Verification items for this drawing (mm, ordinates from the low corner). A direction names the side the tool comes from. Round coordinates to 2 decimals unless told otherwise and drop trailing zeros. Order: outer loops, then holes, each group sorted by start corner. A loop starts at its lowest first (then second) coordinate and runs counter-clockwise, first axis right, second up. Notation, with made-up numbers: (0, -28) - (33, -28) arc R10 ccw to (33, -14) - close; hole circle Ø1 at (-1, 38). An arc over 180 degrees is marked (long way). Return JSON: item names as keys, results as strings. Group by question number.
Q1. Sectioned sample at D-D, the plane x = 1.5. Record the cut outline in (y, z), then the cut area to 3 significant figures.
Q2. Sectioned sample at C-C, the plane y = 5. Record the cut outline in (x, z), then the cut area to 3 significant figures.
Q3. Tool access check on the marked faces 1 and 2. Record the directions out of +Z, -Z, +X, -X, +Y, -Y that give a thin tool (end or side, any length) a straight path to the whole face; none if there is none.
Q4. Material ranges on line 1 along Y through (x, z) = (7.5, 6.5); line 2 along Y through (x, z) = (5.25, 1); line 3 along X through (y, z) = (5, 8), recorded low to high.
Q5. Sectioned sample at A-A, the plane x = 7.5. Record the cut outline in (y, z).
Q6. Sectioned sample at B-B, the plane z = 7.5. Record the cut outline in (x, y), then the cut area to 3 significant figures.
Q7. Gauge pin test, flat ends, axial feed: pin 1 Ø5 at (y, z) = (69.5, 11) entering from -X; pin 2 Ø3.5 at (x, y) = (7.5, 5) entering from +Z; pin 3 Ø2 at (y, z) = (39.5, 9) entering from +X. Record the tip position at first contact, or that the pin passes through.
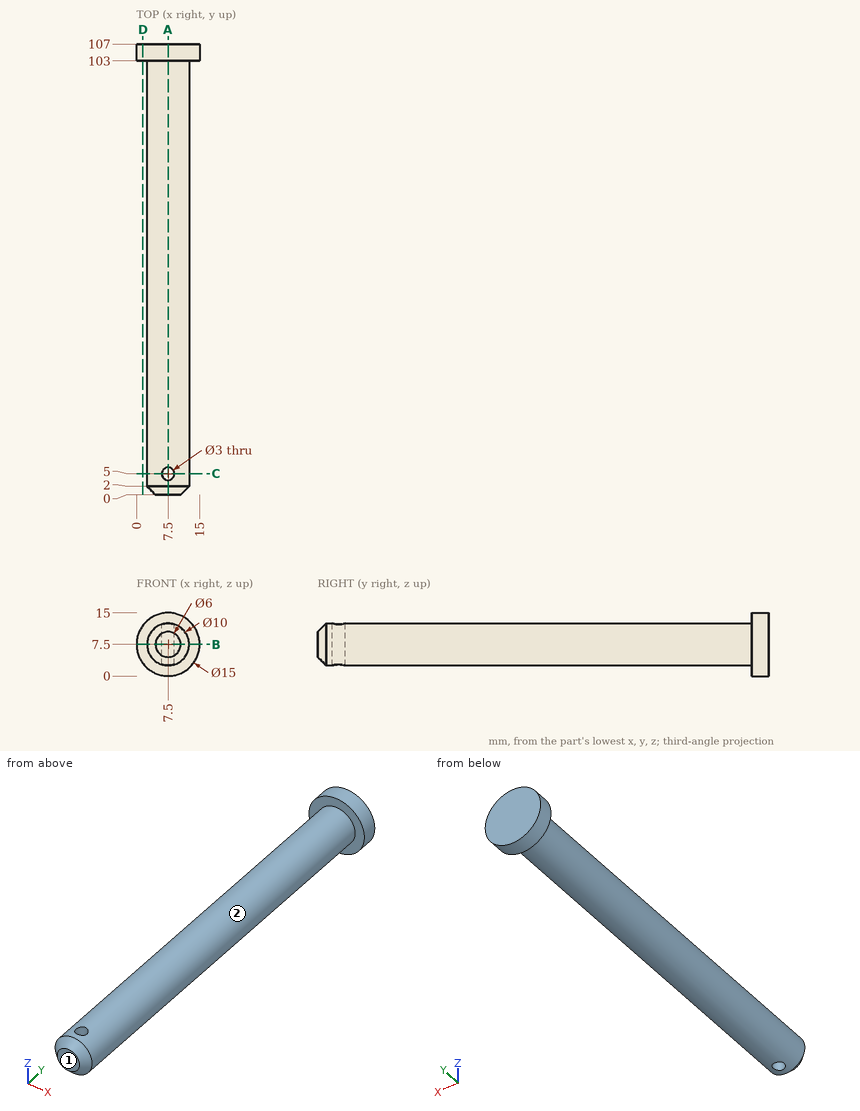
Reply:
{
 "1": {"outline": "(103, 3) - (107, 3) - (107, 12) - (103, 12) - close", "area": "36.0 mm^2"},
 "2": {"outline": "(6, 2.73) - (6, 12.27) arc R5 ccw to start; (9, 2.73) arc R5 ccw to (9, 12.27) - close", "area": "49.0 mm^2"},
 "3": {"face 1": "+Z, -Z, +X, -X, -Y", "face 2": "-Y"},
 "4": {"line 1": "0 to 3.5, 6.5 to 107", "line 2": "103 to 107", "line 3": "2.53 to 6, 9 to 12.47"},
 "5": {"outline": "(0, 4.5) - (2, 2.5) - (3.5, 2.5) - (3.5, 12.5) - (2, 12.5) - (0, 10.5) - close; (6.5, 2.5) - (103, 2.5) - (103, 0) - (107, 0) - (107, 15) - (103, 15) - (103, 12.5) - (6.5, 12.5) - close"},
 "6": {"outline": "(0, 103) - (2.5, 103) - (2.5, 2) - (4.5, 0) - (10.5, 0) - (12.5, 2) - (12.5, 103) - (15, 103) - (15, 107) - (0, 107) - close; hole circle Ø3 at (7.5, 5)", "area": "1,080 mm^2"},
 "7": {"pin 1": "x = 2.6", "pin 2": "z = 12.5", "pin 3": "x = 12.47"}
}
